Design review of the part built by this model. Coordinates are the model's own, in mm. A direction names the side the tool comes from. Coordinates: 2 decimals unless noted, no trailing zeros. Write each loop counter-clockwise with the first axis right and the second up, starting at its lowest first coordinate (ties: lowest second). Pieces come first, ordered by that corner, then holes. Notation, with made-up numbers: (83, 1) -> (136, 1) arc R10 cw to (136, 7) -> close; hole circle Ø4 at (-24.5, 78). An arc over 180 degrees is marked (long way). Return JSON: item names as keys, results as strings. Group by question number.
from build123d import *

# Parameters (mm, degrees)
SKETCH_1_R      = 1.6
SKETCH_1_W      = 3
SKETCH_1_H      = 10
EXTRUDE_1_DEPTH = 3


with BuildPart() as part:
    # 草图1 → 凸台-拉伸1 (new body)
    with BuildSketch(Plane.XY):
        Polygon((32, 0), (44, 0), (56, 0), (56, -3), (76, -3), (76, 0), (88, 0), (91, 0), (91, 30), (88, 30), (0, 30), (-3, 30), (-3, 0), (0, 0), (12, 0), (12, -3), (32, -3), align=None)
        with Locations((30, 4)):
            Circle(SKETCH_1_R, mode=Mode.SUBTRACT)
        Polygon((6, 4), (6, 7), (6, 20), (11, 20), (16, 20), (16, 4), (11, 4), align=None, mode=Mode.SUBTRACT)
        with BuildLine():
            ThreePointArc((59.6, 4), (58, 2.4), (56.4, 4))
            ThreePointArc((56.4, 4), (58, 5.6), (59.6, 4))
        make_face(mode=Mode.SUBTRACT)
        with Locations((78.5, 10)):
            Rectangle(SKETCH_1_W, SKETCH_1_H, mode=Mode.SUBTRACT)
        Polygon((0, 15), (0, 23), (3, 23), (3, 15), (3, 7), (0, 7), align=None, mode=Mode.SUBTRACT)
        Polygon((85, 23), (88, 23), (88, 15), (88, 7), (85, 7), (85, 15), align=None, mode=Mode.SUBTRACT)
    extrude(amount=EXTRUDE_1_DEPTH)


solid = part.part
Q1. We need section B-B on x = 7. Write out the cut boundary in (y, z).
Q2. For P1, Ø0.9, axis at x = 86.5, z = 1.5, coming from the -Y side; P2, Ø1.5, axis at y = -1, z = 2, coming from the -X side, all flat-tipped, find the tip position at first contact; note any pin that passes through.
Q3. We need section A-A on y = 17. Write out the cut boundary in (x, z).
Q4. Wall thickness on L1, parallel to Y at x = 8, z = 1.65; L2, parallel to Y at x = 30, z = 2.15; L3, parallel to X at y = 11, z = 1: over which ranges is each line inside the solid? List them lowest first.
Q5. The part is to be moulded in two halves that separate along X. For faces 4 (the flat face through (3, 15, 1)), 5 (the flat face through (12, -1, 1)), 6 (the flat face through (87, 7, 1)), 7 (the flat face through (45, 30, 1)), say which applies: +X half, -X half, draft (parallel to the pull), parting line (faces both ways), or undercut.
Q6. For faces 1 (the flat face through (78, 5, 1)), 2 (the flat face through (4, 0, 1)), 3 (the flat face through (56, -1, 1)), list the 3-axis set-ups (+Z, -Z, +X, -X, +Y, -Y) from which the entire face can be reached by the end or side of a thin tool; tool diameter is ignored.
Q7. We need section D-D on z = 0.8. State how many separate pieces and enclosed holes the cut face has, plus the area to 3 significant figures.
Q8. We need section C-C on y = 10.5. Write out the cut boundary in (x, z), plus the area to 3 significant figures.
Findings below:
{
 "1": {"outline": "(0, 0) -> (4, 0) -> (4, 3) -> (0, 3) -> close; (20, 0) -> (30, 0) -> (30, 3) -> (20, 3) -> close"},
 "2": {"P1": "stops at y = 0", "P2": "stops at x = 12"},
 "3": {"outline": "(-3, 0) -> (0, 0) -> (0, 3) -> (-3, 3) -> close; (3, 0) -> (6, 0) -> (6, 3) -> (3, 3) -> close; (16, 0) -> (85, 0) -> (85, 3) -> (16, 3) -> close; (88, 0) -> (91, 0) -> (91, 3) -> (88, 3) -> close"},
 "4": {"L1": "y = 0 to 4, 20 to 30", "L2": "y = -3 to 2.4, 5.6 to 30", "L3": "x = -3 to 0, 3 to 6, 16 to 77, 80 to 85, 88 to 91"},
 "5": {"face 4": "undercut", "face 5": "-X half", "face 6": "undercut", "face 7": "draft"},
 "6": {"face 1": "+Z, -Z", "face 2": "+Z, -Z, -X, -Y", "face 3": "+Z, -Z, -Y"},
 "7": {"separate pieces": "1", "enclosed holes": "6", "area": "2,640 mm^2"},
 "8": {"outline": "(-3, 0) -> (0, 0) -> (0, 3) -> (-3, 3) -> close; (3, 0) -> (6, 0) -> (6, 3) -> (3, 3) -> close; (16, 0) -> (77, 0) -> (77, 3) -> (16, 3) -> close; (80, 0) -> (85, 0) -> (85, 3) -> (80, 3) -> close; (88, 0) -> (91, 0) -> (91, 3) -> (88, 3) -> close", "area": "225 mm^2"}
}
